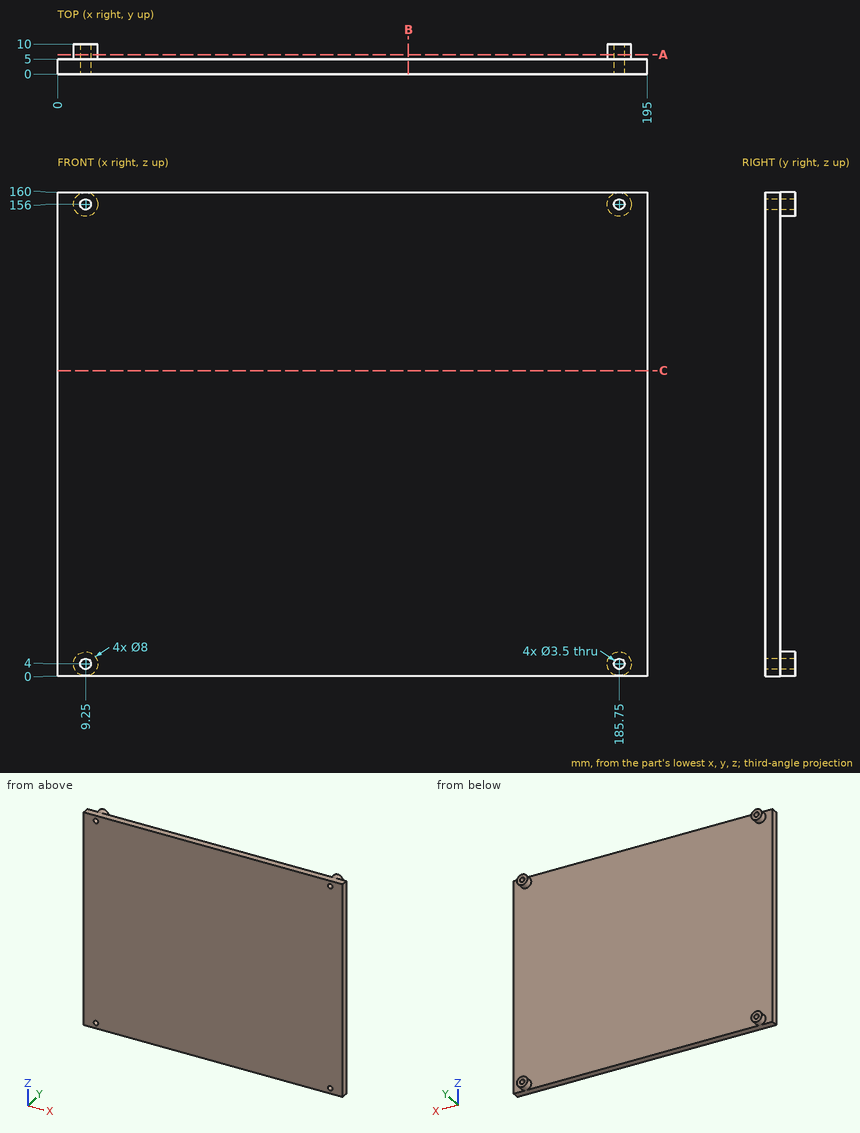
The figure shows three views and two pictorial views of one solid part (mm, origin at its lowest corner). Answer the questions. Coordinates: 2 decimals unless noted, no trailing zeros. Loops run counter-clockwise (first coordinate to the right, second up) from the corner with the lowest first, then second, coordinate; pieces in that order, holes last.
1) Find section C-C on z = 101. Write down the section's boundary in (x, y).
2) Flat-ended cylindrical pins translate along their axes: pin 1 Ø2 at (x, z) = (185.75, 156) entering from +Y; pin 2 Ø2 at (x, z) = (162.5, 38) entering from +Y. Find the tip coordinate at first contact, or state that the pin passes through.
3) Find section B-B on x = 116. Write down the section's boundary in (y, z), then the cut area to 3 significant figures.
4) Find section A-A on y = 6.5. Write down the section's boundary in (x, z).
5) Find the intervals of material crossed by L1, parallel to X at y = 4, z = 156; L2, parallel to X at y = 6.5, z = 4; L3, parallel to Z at x = 185.75, y = 3, in increasing order.
Values:
1. outline: (0, 0) - (195, 0) - (195, 5) - (0, 5) - close
2. pin 1: passes through
2. pin 2: stops at y = 5
3. outline: (0, 0) - (5, 0) - (5, 160) - (0, 160) - close
3. area: 800 mm2
4. outline: circle Ø8 at (9.25, 4); circle Ø8 at (9.25, 156); circle Ø8 at (185.75, 4); circle Ø8 at (185.75, 156); hole circle Ø3.5 at (9.25, 4); hole circle Ø3.5 at (9.25, 156); hole circle Ø3.5 at (185.75, 4); hole circle Ø3.5 at (185.75, 156)
5. L1: x = 0 to 7.5, 11 to 184, 187.5 to 195
5. L2: x = 5.25 to 7.5, 11 to 13.25, 181.75 to 184, 187.5 to 189.75
5. L3: z = 0 to 2.25, 5.75 to 154.25, 157.75 to 160
